Part model, mm, in its own coordinate system. Face numbers are marked on the shaded views. Coordinates: 2 decimals unless noted, no trailing zeros. Loops run counter-clockwise (first coordinate to the right, second up) from the corner with the lowest first, then second, coordinate; pieces in that order, holes last.
```python
from build123d import *

# Parameters (mm, degrees)
SKETCH2_R           = 20
SKETCH3_W           = 40
SKETCH3_H           = 40
BOSS_EXTRUDE1_DEPTH = 225
CIRPATTERN1_COUNT   = 4
SKETCH8_R           = 337
SKETCH8_R_2         = 273
BOSS_EXTRUDE3_DEPTH = 20
BOSS_EXTRUDE4_DEPTH = 20
SKETCH12_W          = 60
SKETCH12_H          = 50
SKETCH12_W_2        = 50
SKETCH12_H_2        = 60
BOSS_EXTRUDE5_DEPTH = 20


with BuildPart() as part:
    # Sketch2 → Revolve1 (revolve)
    with BuildSketch(Plane.XY, mode=Mode.PRIVATE) as revolve1_sk:
        with Locations((300, 0)):
            Circle(SKETCH2_R)
    revolve(revolve1_sk.sketch.rotate(Axis((0, 0, 0), (0, 1, 0)), 90), axis=Axis((0, 0, 0), (0, 1, 0)))

    # Sketch3 → Boss-Extrude1 (add)
    with BuildSketch(Plane.XY.offset(300)):
        Rectangle(SKETCH3_W, SKETCH3_H)
    boss_extrude1 = extrude(amount=-BOSS_EXTRUDE1_DEPTH)

    # CirPattern1: Boss-Extrude1 ×4 about axis
    cirpattern1_axis = Axis((0, 0, 0), (0, 1, 0))
    for i in range(1, CIRPATTERN1_COUNT):
        add(boss_extrude1.rotate(cirpattern1_axis, i * 360 / CIRPATTERN1_COUNT))

    # Sketch8 → Boss-Extrude3 (add, symmetric)
    with BuildSketch(Plane(origin=(0, 0, 0), x_dir=(1, 0, 0), z_dir=(0, 1, 0))):
        with Locations(Location((0, 0, 0), (0, 0, 270))):
            Circle(SKETCH8_R)
        Circle(SKETCH8_R_2, mode=Mode.SUBTRACT)
    extrude(amount=BOSS_EXTRUDE3_DEPTH, both=True)

    # Sketch9 → Boss-Extrude4 (add, symmetric)
    with BuildSketch(Plane(origin=(0, 0, 0), x_dir=(1, 0, 0), z_dir=(0, 1, 0))):
        with BuildLine():
            Line((-20, -75), (-20, -72.284161474))
            ThreePointArc((-20, -72.284161474), (-53.033008589, -53.033008589), (-72.284161474, -20))
            Line((-72.284161474, -20), (-75, -20))
            Line((-75, -20), (-75, 20))
            Line((-75, 20), (-72.284161474, 20))
            ThreePointArc((-72.284161474, 20), (-53.033008589, 53.033008589), (-20, 72.284161474))
            Line((-20, 72.284161474), (-20, 75))
            Line((-20, 75), (20, 75))
            Line((20, 75), (20, 72.284161474))
            ThreePointArc((20, 72.284161474), (53.033008589, 53.033008589), (72.284161474, 20))
            Line((72.284161474, 20), (75, 20))
            Line((75, 20), (75, -20))
            Line((75, -20), (72.284161474, -20))
            ThreePointArc((72.284161474, -20), (53.033008589, -53.033008589), (20, -72.284161474))
            Line((20, -72.284161474), (20, -75))
            Line((20, -75), (-20, -75))
        make_face()
    extrude(amount=BOSS_EXTRUDE4_DEPTH, both=True)

    # Sketch12 → Boss-Extrude5 (add)
    with BuildSketch(Plane(origin=(0, 20, 0), x_dir=(1, 0, 0), z_dir=(0, 1, 0))):
        with Locations((305, 0)):
            Rectangle(SKETCH12_W, SKETCH12_H)
        with Locations((0, -305)):
            Rectangle(SKETCH12_W_2, SKETCH12_H_2)
        with Locations((-305, 0)):
            Rectangle(SKETCH12_W, SKETCH12_H)
        with Locations((0, 305)):
            Rectangle(SKETCH12_W_2, SKETCH12_H_2)
    extrude(amount=BOSS_EXTRUDE5_DEPTH)


solid = part.part
```
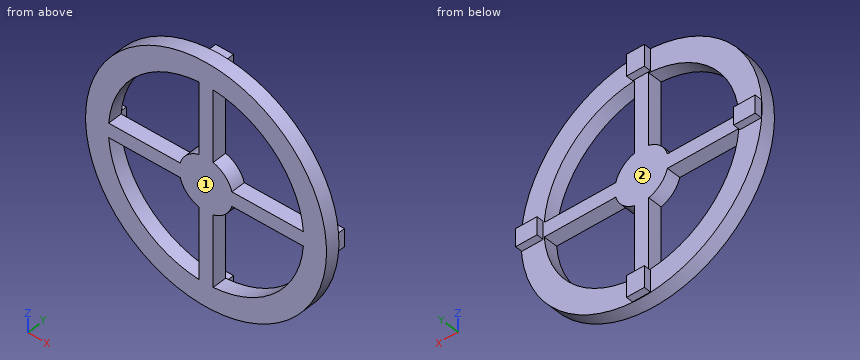
Q1. Probe line 1 (X direction, y = -13, z = 152.5); line 2 (Z direction, x = -45, y = 12); line 3 (Z direction, x = 109, y = 16). List the from-to ranges inside material, lowest first.
Q2. Saw through at B-B (x = 0). List the corners of the cut face in (y, z), plus the area to 3 significant figures.
Q3. Drop flat-ended pins along their axis: P1, Ø16, axis at y = 33.5, z = 308.5, coming from the +X side; P2, Ø10, axis at y = 12, z = 251, coming from the +X side; P3, Ø6, axis at x = 307, y = 27, coming from the +Z side. Give the stop position or say it passes through.
Q4. Saw through at C-C (z = -43). List the corners of the cut face in (x, y), plus the area to 3 significant figures.
Q5. Mould opens along Z. For the marked faces 1 and 2 say: released by +Z, released by -Z, zero draft, split by the parting line, or undercut.
Q6. Saw through at D-D (x = -228). List the corners of the cut face in (y, z).
Q7. Saw through at A-A (y = 3). List the corners of the cut face in (x, z), plus the area to 3 significant figures.
Checked values:
1. line 1: x = -300.52 to -226.43, -20 to 20, 226.43 to 300.52
1. line 2: z = -333.98 to -269.27, -60 to 60, 269.27 to 333.98
1. line 3: z = -318.89 to -250.3, -20 to 20, 250.3 to 318.89
2. outline: (-20, -337) - (20, -337) - (20, -335) - (40, -335) - (40, -275) - (20, -275) - (20, 275) - (40, 275) - (40, 335) - (20, 335) - (20, 337) - (-20, 337) - close
2. area: 29,400 mm2
3. P1: stops at x = 25
3. P2: stops at x = 230.33
3. P3: stops at z = 25
4. outline: (-334.25, -20) - (-269.59, -20) - (-269.59, 20) - (-334.25, 20) - close; (-61.45, -20) - (61.45, -20) - (61.45, 20) - (-61.45, 20) - close; (269.59, -20) - (334.25, -20) - (334.25, 20) - (269.59, 20) - close
4. area: 10,100 mm2
5. face 1: zero draft
5. face 2: undercut
6. outline: (-20, -248.16) - (20, -248.16) - (20, -150.15) - (-20, -150.15) - close; (-20, -20) - (20, -20) - (20, 20) - (-20, 20) - close; (-20, 150.15) - (20, 150.15) - (20, 248.16) - (-20, 248.16) - close
7. outline: circle Ø674 at (0, 0); hole (-272.27, -20) arc R273 ccw to (-20, -272.27) - (-20, -72.28) arc R75 cw to (-72.28, -20) - close; hole (-272.27, 20) - (-72.28, 20) arc R75 cw to (-20, 72.28) - (-20, 272.27) arc R273 ccw to start; hole (20, -272.27) arc R273 ccw to (272.27, -20) - (72.28, -20) arc R75 cw to (20, -72.28) - close; hole (20, 72.28) arc R75 cw to (72.28, 20) - (272.27, 20) arc R273 ccw to (20, 272.27) - close
7. area: 172,000 mm2
